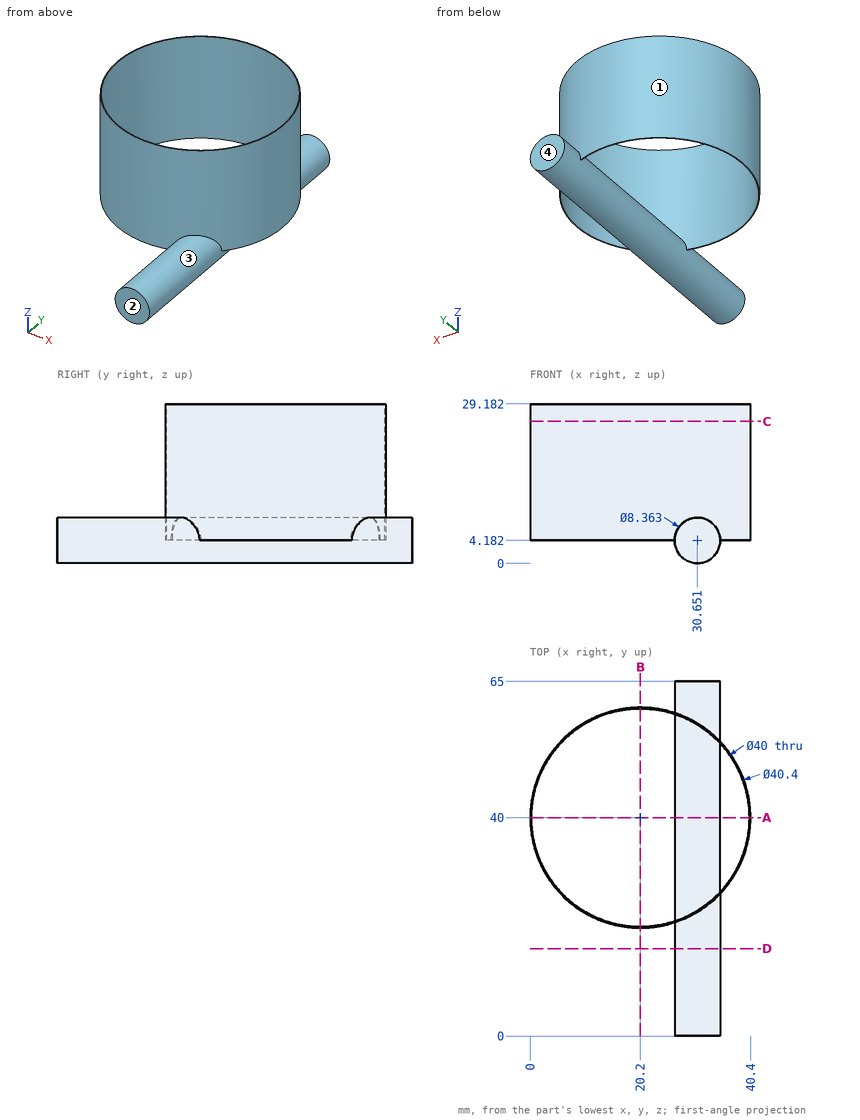
Verification items for this drawing (mm, ordinates from the low corner). A direction names the side the tool comes from. Coordinates: 2 decimals unless noted, no trailing zeros. Loops run counter-clockwise (first coordinate to the right, second up) from the corner with the lowest first, then second, coordinate; pieces in that order, holes last. Notation, with made-up numbers: (85.5, 51) - (112.5, 51) arc R35 ccw to (112.5, 87) - close; hole circle Ø9 at (5.5, 37.5). An arc over 180 degrees is marked (long way). Use one line per item in the form item = value. Start each with the question number.
Item 1: Section check B-B, the plane x = 20.2. Enter the section's corners in (y, z).
Item 2: Section check C-C, the plane z = 26. Enter the section's corners in (x, y).
Item 3: Section check A-A, the plane y = 40. Enter the section's corners in (x, z).
Item 4: Section check D-D, the plane y = 16. Enter the section's corners in (x, z).
Item 5: Thickness scan on probe 1 along Y at (x, z) = (20.2, 16.5); probe 2 along X at (y, z) = (48.5, 8.75) (1 decimal); probe 3 along X at (y, z) = (48, 11). Record the ranges inside material, lowest first.
Item 6: Gauge pin test, flat ends, axial feed: pin 1 (5 mm diameter, centred on x = 10.5, z = 5, fed in from -Y); pin 2 (1.5 mm diameter, centred on y = 58, z = 17.5, fed in from +X); pin 3 (3 mm diameter, centred on x = 38.5, y = 33, fed in from -Z). Record the tip position at first contact, or that the pin passes through.
Item 7: Mould release check, pull along X, two halves, no side actions. Record for the marked faces 3 and 4: +X half, -X half, draft (parallel to the pull), parting line (faces both ways), or undercut.
Item 8: Tool access check on the marked faces 1 and 2. Record the directions out of +Z, -Z, +X, -X, +Y, -Y that give a thin tool (end or side, any length) a straight path to the whole face; none if there is none.
Computed:
q1.outline = (19.8, 4.18) - (20, 4.18) - (20, 29.18) - (19.8, 29.18) - close; (60, 4.18) - (60.2, 4.18) - (60.2, 29.18) - (60, 29.18) - close
q2.outline = circle Ø40.4 at (20.2, 40); hole circle Ø40 at (20.2, 40)
q3.outline = (0, 4.18) - (0.2, 4.18) - (0.2, 29.18) - (0, 29.18) - close; circle Ø8.36 at (30.65, 4.18); (40.2, 4.18) - (40.4, 4.18) - (40.4, 29.18) - (40.2, 29.18) - close
q4.outline = circle Ø8.36 at (30.65, 4.18)
q5.probe_1 = 19.8 to 20, 60 to 60.2
q5.probe_2 = 1.9 to 2.1, 38.3 to 38.5
q5.probe_3 = 1.65 to 1.87, 38.53 to 38.75
q6.pin_1 = 21.13
q6.pin_2 = 30.71
q6.pin_3 = 4.18
q7.face_3 = undercut
q7.face_4 = draft
q8.face_1 = +Z
q8.face_2 = +Z, -Z, +X, -X, -Y
